from build123d import *

# Parameters (mm, degrees)
SKETCH1_W             = 9.525
SKETCH1_H             = 76.2
BOSS_EXTRUDE1_DEPTH   = 165.1
F_8_CLEARANCE_HOLE1_D = 4.4958
F_8_CLEARANCE_HOLE2_D = 4.4958


with BuildPart() as part:
    # Sketch1 → Boss-Extrude1 (new body)
    with BuildSketch(Plane.XY):
        Rectangle(SKETCH1_W, SKETCH1_H)
    extrude(amount=BOSS_EXTRUDE1_DEPTH)

    # #8 Clearance Hole1 (through all)
    with Locations(Plane(origin=(4.7625, 0, 0), x_dir=(0, 0, -1), z_dir=(1, 0, 0))):
        with Locations((-52.3875, -30.1625), (-112.7125, 30.1625), (-112.7125, -30.1625), (-52.3875, 30.1625)):
            Hole(F_8_CLEARANCE_HOLE1_D / 2)

    # #8 Clearance Hole2 (through all)
    with Locations(Plane(origin=(4.7625, 0, 0), x_dir=(0, 0, -1), z_dir=(1, 0, 0))):
        with Locations((-152.4, 25.4), (-152.4, 0), (-152.4, -25.4), (-12.7, 25.4), (-12.7, 0), (-12.7, -25.4)):
            Hole(F_8_CLEARANCE_HOLE2_D / 2)


solid = part.part
Model file for the job. Use its own axes, mm. Give positions to 0.01 mm unless a question says otherwise; leave off trailing zeros. Loops run counter-clockwise (first coordinate to the right, second up) from the corner with the lowest first, then second, coordinate; pieces in that order, holes last.
1) Saw through at B-B (y = -25.4). Write the cut outline in (x, z).
2) Wall check: line 1 (Y direction, x = 2.25, z = 152.4); line 2 (Z direction, x = -0.5, y = -26); line 3 (Y direction, x = -1, z = 111.5). Give the ranges that are in metal, low to high.
3) Flat gauge pin, fed straight in: pin 1 Ø5 at (y, z) = (30.16, 52.39) entering from -X. Where does the tip first touch, or does it go through?
4) Saw through at A-A (z = 152.4). Write the cut outline in (x, y).
5) Pull direction Y, two halves, no side cores. Call faces 1 (the flat face through (0, 1, 0)), 2 (the cylindrical face through (-0.067, 0.099, 150.154)), 3 (the cylindrical face through (-0.067, 30.261, 110.467)), 4 (the flat face through (0, -38.1, 81)): +Y half, -Y half, draft (parallel to the pull), parting line (faces both ways), or undercut.
6) Saw through at C-C (z = 113.5). Write the cut outline in (x, y).
Answer block:
1. outline: (-4.76, 0) - (4.76, 0) - (4.76, 10.45) - (-4.76, 10.45) - close; (-4.76, 14.95) - (4.76, 14.95) - (4.76, 150.15) - (-4.76, 150.15) - close; (-4.76, 154.65) - (4.76, 154.65) - (4.76, 165.1) - (-4.76, 165.1) - close
2. line 1: y = -38.1 to -27.65, -23.15 to -2.25, 2.25 to 23.15, 27.65 to 38.1
2. line 2: z = 0 to 10.53, 14.87 to 150.23, 154.57 to 165.1
2. line 3: y = -38.1 to -32.06, -28.27 to 28.27, 32.06 to 38.1
3. pin 1: stops at x = -4.76
4. outline: (-4.76, -38.1) - (4.76, -38.1) - (4.76, -27.65) - (-4.76, -27.65) - close; (-4.76, -23.15) - (4.76, -23.15) - (4.76, -2.25) - (-4.76, -2.25) - close; (-4.76, 2.25) - (4.76, 2.25) - (4.76, 23.15) - (-4.76, 23.15) - close; (-4.76, 27.65) - (4.76, 27.65) - (4.76, 38.1) - (-4.76, 38.1) - close
5. face 1: draft
5. face 2: undercut
5. face 3: undercut
5. face 4: -Y half
6. outline: (-4.76, -38.1) - (4.76, -38.1) - (4.76, -32.27) - (-4.76, -32.27) - close; (-4.76, -28.06) - (4.76, -28.06) - (4.76, 28.06) - (-4.76, 28.06) - close; (-4.76, 32.27) - (4.76, 32.27) - (4.76, 38.1) - (-4.76, 38.1) - close
